Check sheet for the modelled part. Datum: model origin and axes. Units: mm. A direction names the side the tool comes from. Round coordinates to 2 decimals unless told otherwise and drop trailing zeros. Write each loop counter-clockwise with the first axis right and the second up, starting at its lowest first coordinate (ties: lowest second). Pieces come first, ordered by that corner, then holes. Notation, with made-up numbers: M -1,78.25 L 56,78.25 A16 ccw 56,108.25 Z; hole C 18.25,15 d2. An arc over 180 degrees is marked long. Answer in a Markdown table with one row per item.
```python
from build123d import *

# Parameters (mm, degrees)
F0_R     = 5.275
F0_R_2   = 5.75
F0_R_3   = 7.5
F0_R_4   = 6.875
F1_DEPTH = 12.85
F2_R     = 44.65
F2_R_2   = 41.275
F3_DEPTH = 1.91
F4_R     = 2.2
F5_DEPTH = 7


with BuildPart() as f1:
    # F0 (on Top) → F1 (new body)
    with BuildSketch(Plane.XY):
        with BuildLine():
            ThreePointArc((63.45, 57.65), (61.8390872965, 61.5390872965), (57.95, 63.15))
            Line((57.95, 63.15), (-57.95, 63.15))
            ThreePointArc((-57.95, 63.15), (-61.8390872965, 61.5390872965), (-63.45, 57.65))
            Line((-63.45, 57.65), (-63.45, -57.65))
            ThreePointArc((-63.45, -57.65), (-61.8390872965, -61.5390872965), (-57.95, -63.15))
            Line((-57.95, -63.15), (57.95, -63.15))
            ThreePointArc((57.95, -63.15), (61.8390872965, -61.5390872965), (63.45, -57.65))
            Line((63.45, -57.65), (63.45, 57.65))
        make_face()
        with Locations((-54.725, -52.975)):
            Circle(F0_R, mode=Mode.SUBTRACT)
        with Locations((52.525, -53.875)):
            Circle(F0_R, mode=Mode.SUBTRACT)
        with Locations((0.2, -0.2)):
            Circle(F0_R_2, mode=Mode.SUBTRACT)
        with Locations((-28.2, 0.45)):
            Circle(F0_R_3, mode=Mode.SUBTRACT)
        with Locations((-53.425, 53.875)):
            Circle(F0_R, mode=Mode.SUBTRACT)
        with Locations((24.675, 1.225)):
            Circle(F0_R_4, mode=Mode.SUBTRACT)
        with Locations((53.175, 52.825)):
            Circle(F0_R, mode=Mode.SUBTRACT)
    extrude(amount=F1_DEPTH)

    # F2 (on face) → F3 (cut)
    with BuildSketch(Plane(origin=(0, 0, 0), x_dir=(1, 0, 0), z_dir=(0, 0, -1))):
        with Locations((0.1, -0.6)):
            Circle(F2_R)
        with Locations((0.1, -0.6)):
            Circle(F2_R_2, mode=Mode.SUBTRACT)
    extrude(amount=-F3_DEPTH, mode=Mode.SUBTRACT)

    # F4 (on face) → F5 (cut)
    with BuildSketch(Plane.XY.offset(12.85)):
        with Locations((-21.46, 12.124022443)):
            Circle(F4_R)
        with Locations((-34.94, 12.124022443)):
            Circle(F4_R)
        with Locations((-41.68, 0.45)):
            Circle(F4_R)
        with Locations((-34.94, -11.224022443)):
            Circle(F4_R)
        with Locations((-21.46, -11.224022443)):
            Circle(F4_R)
        with Locations((-14.72, 0.45)):
            Circle(F4_R)
    extrude(amount=-F5_DEPTH, mode=Mode.SUBTRACT)


solid = f1.part
```
1. Section check D-D, the plane z = 11.25. Count the separate pieces of the cut face and the enclosed holes in it, and give its area (3 significant figures).
Found:
| item | result |
|---|---|
| separate pieces | 1 |
| enclosed holes | 13 |
| area | 15,100 mm2 |
2. Go/stop test with flat-tipped pins: pin 1 (5 mm diameter, centred on x = -34.94, y = 12.12, fed in from +Z); pin 2 (9.5 mm diameter, centred on x = 53.175, y = 52.825, fed in from -Z); pin 3 (1.3 mm diameter, centred on x = -34, y = -10.5, fed in from +Z). Record where each tip stops, or that it passes through.
Found:
| item | result |
|---|---|
| pin 1 | stops at z = 12.85 |
| pin 2 | passes through |
| pin 3 | stops at z = 5.85 |
3. Section check C-C, the plane z = 3.5. Record the cut outline in (x, y) (3 decimals), and give its area (3 significant figures).
Found:
| item | result |
|---|---|
| outline | M -63.45,-57.65 A5.5 ccw -57.95,-63.15 L 57.95,-63.15 A5.5 ccw 63.45,-57.65 L 63.45,57.65 A5.5 ccw 57.95,63.15 L -57.95,63.15 A5.5 ccw -63.45,57.65 Z; hole C -54.725,-52.975 d10.55; hole C -53.425,53.875 d10.55; hole C -28.2,0.45 d15; hole C 0.2,-0.2 d11.5; hole C 24.675,1.225 d13.75; hole C 52.525,-53.875 d10.55; hole C 53.175,52.825 d10.55 |
| area | 15,200 mm2 |
4. Section check A-A, the plane x = -54.5. Record the cut outline in (y, z), and give its area (3 significant figures).
Found:
| item | result |
|---|---|
| outline | M -63.15,0 L -58.25,0 L -58.25,12.85 L -63.15,12.85 Z; M -47.7,0 L 48.71,0 L 48.71,12.85 L -47.7,12.85 Z; M 59.04,0 L 63.15,0 L 63.15,12.85 L 59.04,12.85 Z |
| area | 1,350 mm2 |
5. Scan lines: L1, parallel to X at y = -53.5, z = 6.5; L2, parallel to Y at x = -14.72, z = 9; L3, parallel to Y at x = 54, z = 8.5. Record each from-to range of solid material in increasing order.
Found:
| item | result |
|---|---|
| L1 | x = -63.45 to -59.97, -49.48 to 47.26, 57.79 to 63.45 |
| L2 | y = -63.15 to -1.75, 2.65 to 63.15 |
| L3 | y = -63.15 to -58.94, -48.81 to 47.61, 58.04 to 63.15 |
6. Section check B-B, the plane y = 50.5. Record the cut outline in (x, z), and give its area (3 significant figures).
Found:
| item | result |
|---|---|
| outline | M -63.45,0 L -57.48,0 L -57.48,12.85 L -63.45,12.85 Z; M -49.37,0 L 48.44,0 L 48.44,12.85 L -49.37,12.85 Z; M 57.91,0 L 63.45,0 L 63.45,12.85 L 57.91,12.85 Z |
| area | 1,400 mm2 |
7. Draft check along Y on faces 1 (the face through (13, 1, 12.85)), 2 (the face through (-1, -63.15, 6)), 3 (the face through (-20.445, 10.172, 9.399)). Enter one of: +Y half, -Y half, draft (parallel to the pull), parting line (faces both ways), or undercut.
Found:
| item | result |
|---|---|
| face 1 | draft |
| face 2 | -Y half |
| face 3 | undercut |
8. Access from +Z, -Z, +X, -X, +Y, -Y to the whole of each face (thin tool, end or side, straight path). Record for faces 4 (the face through (-9.58, 44.19, 0.94)), 5 (the face through (-52.291, -57.655, 6.335)), 6 (the face through (-16.918, 0.547, 9.399)).
Found:
| item | result |
|---|---|
| face 4 | -Z |
| face 5 | +Z, -Z |
| face 6 | +Z |
